from build123d import *

# Parameters (mm, degrees)
SZKIC1_R                    = 2.5
SZKIC1_R_2                  = 1.5
DODANIE_WYCI_GNI_CIE1_DEPTH = 10


with BuildPart() as part:
    # Szkic1 → Dodanie-wyciągnięcie1 (new body)
    with BuildSketch(Plane(origin=(0, 0, 0), x_dir=(0, 0, -1), z_dir=(1, 0, 0))):
        with BuildLine():
            Line((-20, 4.5), (20, 4.5))
            Line((20, 4.5), (20, -0.5))
            Line((20, -0.5), (4.472135955, -0.5))
            ThreePointArc((4.472135955, -0.5), (0, -4.5), (-4.472135955, -0.5))
            Line((-4.472135955, -0.5), (-20, -0.5))
            Line((-20, -0.5), (-20, 4.5))
        make_face()
        Circle(SZKIC1_R, mode=Mode.SUBTRACT)
        with Locations((17, 2)):
            Circle(SZKIC1_R_2, mode=Mode.SUBTRACT)
        with Locations(Location((-17, 2, 0), (0, 0, 180))):
            Circle(SZKIC1_R_2, mode=Mode.SUBTRACT)
    extrude(amount=DODANIE_WYCI_GNI_CIE1_DEPTH)


solid = part.part
Input: part model. Units: mm. Frame: model coordinates. A direction names the side the tool comes from. Coordinates: 2 decimals unless noted, no trailing zeros. Loops run counter-clockwise (first coordinate to the right, second up) from the corner with the lowest first, then second, coordinate; pieces in that order, holes last. Notation, with made-up numbers: (79, 67.25) - (125, 67.25) arc R15 cw to (125, 78.25) - close; hole circle Ø11 at (-23, -18.75). An arc over 180 degrees is marked (long way). Answer in a Markdown table with one row per item. Add a question column.
Item 1: Line query: line 1 along Y through (x, z) = (4, 17); line 2 along Z through (x, y) = (3.5, 3.25); line 3 along Z through (x, y) = (4.75, 1.75). Output: solid intervals per line, ascending. Write a range as [from, to].
Item 2: Section query C-C on y = 0. Return the cut outline in (x, z).
Item 3: Contact query for flat-ended pins moving along their axis: P1, Ø2.5, axis at y = 2, z = -17, coming from the +X side; P2, Ø4, axis at x = 9, z = -15, coming from the -Y side. Output: stop coordinate, or through.
Item 4: Section query B-B on x = 4.5. Return the cut outline in (y, z), then the cut area to 3 significant figures.
Item 5: Section query A-A on z = 0. Return the cut outline in (x, y), then the cut area to 3 significant figures.
Item 6: Access query for faces 1 (the cylindrical face through (4.93, 2.07, -15.5)), 2 (the flat face through (5, -0.5, -12)). Directions: +Z, -Z, +X, -X, +Y, -Y. A direction counts if a zero-diameter tool reaches every point of the face in a straight line with its end or side. Return the directions, or none.
Item 7: Section query D-D on z = 10.5. Return the cut outline in (x, y), then the cut area to 3 significant figures.
Item 8: Mould query, pull axis Y, two halves, no side actions, for faces 3 (the cylindrical face through (4.93, 1.93, 15.5)), 4 (the flat face through (0, 3, 0)), 5 (the flat face through (5, -0.5, 12)). Classes: released by +Y, released by -Y, zero draft, split by the parting line, or undercut.
Recorded:
| question | item | result |
|---|---|---|
| 1 | line 1 | [-0.5, 0.5], [3.5, 4.5] |
| 1 | line 2 | [-20, -17.83], [-16.17, 16.17], [17.83, 20] |
| 1 | line 3 | [-20, -18.48], [-15.52, -1.79], [1.79, 15.52], [18.48, 20] |
| 2 | outline | (0, -20) - (10, -20) - (10, -2.5) - (0, -2.5) - close; (0, 2.5) - (10, 2.5) - (10, 20) - (0, 20) - close |
| 3 | P1 | through |
| 3 | P2 | y = -0.5 |
| 4 | outline | (-0.5, -20) - (4.5, -20) - (4.5, 20) - (-0.5, 20) - (-0.5, 4.47) arc R4.5 ccw to (-0.5, -4.47) - close; hole circle Ø5 at (0, 0); hole circle Ø3 at (2, -17); hole circle Ø3 at (2, 17) |
| 4 | area | 194 mm^2 |
| 5 | outline | (0, -4.5) - (10, -4.5) - (10, -2.5) - (0, -2.5) - close; (0, 2.5) - (10, 2.5) - (10, 4.5) - (0, 4.5) - close |
| 5 | area | 40.0 mm^2 |
| 6 | face 1 | +X, -X |
| 6 | face 2 | -Z, +X, -X, -Y |
| 7 | outline | (0, -0.5) - (10, -0.5) - (10, 4.5) - (0, 4.5) - close |
| 7 | area | 50.0 mm^2 |
| 8 | face 3 | undercut |
| 8 | face 4 | zero draft |
| 8 | face 5 | released by -Y |
